For this review, use the dimensioned drawing (mm, ordinates from the lowest corner) and the shaded views. A direction names the side the tool comes from. Round coordinates to 2 decimals unless told otherwise and drop trailing zeros. Loops run counter-clockwise (first coordinate to the right, second up) from the corner with the lowest first, then second, coordinate; pieces in that order, holes last. Notation, with made-up numbers: M 46.5,-20 L 73.5,-20 A14 ccw 73.5,-1 Z; hole C -24,5 d2. An arc over 180 degrees is marked long. Use a Markdown table: item, result. Add a question column.
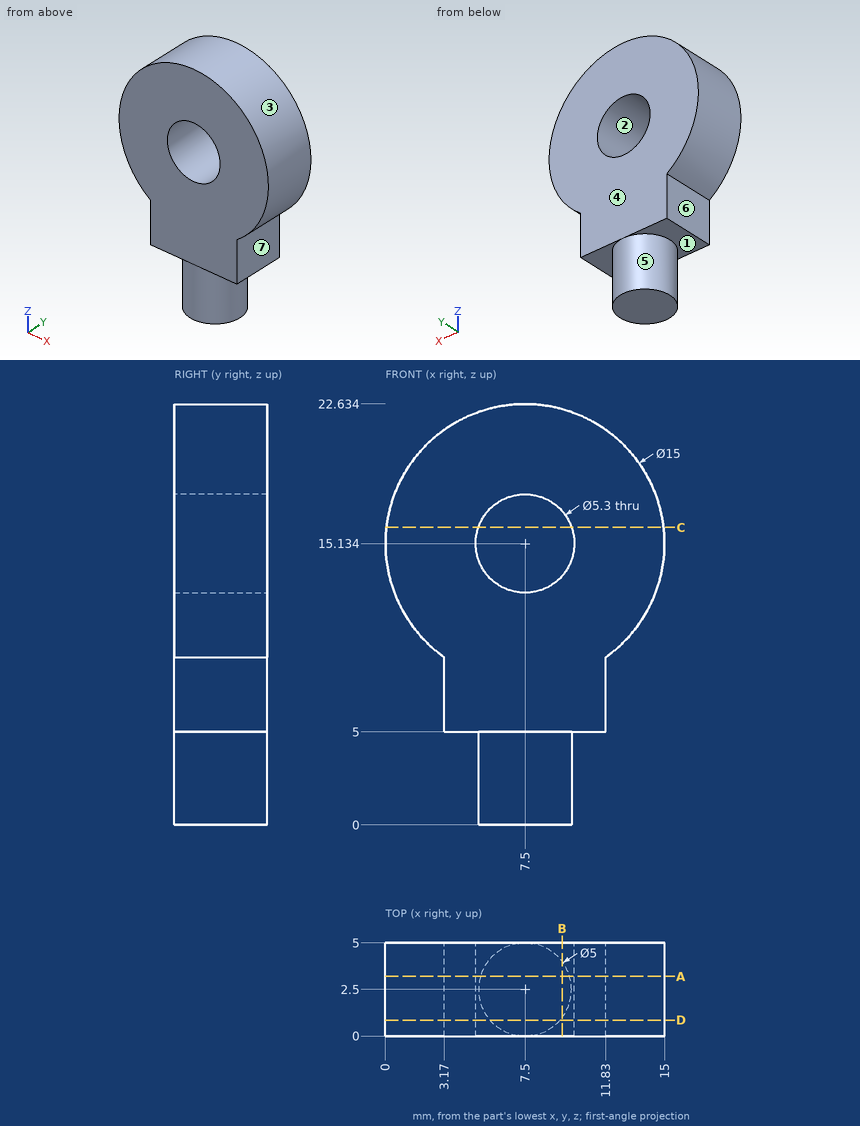
(1) For the marked faces 5, 6 and 7, list the 3-axis set-ups (+Z, -Z, +X, -X, +Y, -Y) from which the entire face can be reached by the end or side of a thin tool; tool diameter is ignored.
(2) Consider section C-C, the plane z = 16. Give the boundary of the cut face in (x, y).
(3) Consider section B-B, the plane x = 9.5. Give the boundary of the cut face in (y, z), then the cut area to 3 significant figures.
(4) Consider section A-A, the plane y = 3.2. Give the boundary of the cut face in (x, z), then the cut area to 3 significant figures.
(5) To check wall thickness, follow probe 1 along X at (y, z) = (4, 16.25); probe 2 along X at (y, z) = (3.3, 6); probe 3 along X at (y, z) = (4.7, 17.25) (1 decimal). State the ranges of each line that lie inside material, in increasing order.
(6) Consider section D-D, the plane y = 0.85. Give the boundary of the cut face in (x, z).
(7) Draft analysis for pull direction Z (two halves, no side actions). For the marked faces 1, 2, 3 and 4, state which applies: released by +Z, released by -Z, zero draft, split by the parting line, or undercut.
(8) Insertion check: pin 1 Ø2 at (y, z) = (2.5, 7) entering from +X; pin 2 Ø3 at (x, y) = (11, 4.5) entering from +Z; pin 3 Ø2 at (y, z) = (2.5, 7) entering from -X. Each pin has a flat end and moves straight along its axis. Give the tip position at first contact, or say it passes through.
Found:
| question | item | result |
|---|---|---|
| 1 | face 5 | -Z |
| 1 | face 6 | -Z, -X, +Y, -Y |
| 1 | face 7 | -Z, +X, +Y, -Y |
| 2 | outline | M 0.05,0 L 5,0 L 5,5 L 0.05,5 Z; M 10,0 L 14.95,0 L 14.95,5 L 10,5 Z |
| 3 | outline | M 0,5 L 1,5 L 1,0 L 4,0 L 4,5 L 5,5 L 5,13.4 L 0,13.4 Z; M 0,16.87 L 5,16.87 L 5,22.36 L 0,22.36 Z |
| 3 | area | 84.4 mm^2 |
| 4 | outline | M 3.17,5 L 5.1,5 L 5.1,0 L 9.9,0 L 9.9,5 L 11.83,5 L 11.83,9.01 A7.5 ccw long 3.17,9.01 Z; hole C 7.5,15.13 d5.3 |
| 4 | area | 205 mm^2 |
| 5 | probe 1 | x = 0.08 to 5.1, 9.9 to 14.92 |
| 5 | probe 2 | x = 3.17 to 11.83 |
| 5 | probe 3 | x = 0.3 to 5.9, 9.1 to 14.7 |
| 6 | outline | M 3.17,5 L 5.62,5 L 5.62,0 L 9.38,0 L 9.38,5 L 11.83,5 L 11.83,9.01 A7.5 ccw long 3.17,9.01 Z; hole C 7.5,15.13 d5.3 |
| 7 | face 1 | released by -Z |
| 7 | face 2 | undercut |
| 7 | face 3 | split by the parting line |
| 7 | face 4 | zero draft |
| 8 | pin 1 | stops at x = 11.83 |
| 8 | pin 2 | stops at z = 22.36 |
| 8 | pin 3 | stops at x = 3.17 |
